```python
from build123d import *

# Parameters (mm, degrees)
SKETCH1_R           = 40
SKETCH1_R_2         = 25
BOSS_EXTRUDE1_DEPTH = 50
SKETCH2_R           = 2
CUT_EXTRUDE1_DEPTH  = 10
BOSS_EXTRUDE2_START = -30
BOSS_EXTRUDE2_DEPTH = 50


with BuildPart() as part:
    # Sketch1 → Boss-Extrude1 (new, symmetric)
    with BuildSketch(Plane(origin=(0, 0, 0), x_dir=(1, 0, 0), z_dir=(0, 1, 0))):
        with Locations(Location((0, 0, 0), (0, 0, 90))):
            Circle(SKETCH1_R)
        with Locations(Location((0, 0, 0), (0, 0, 90))):
            Circle(SKETCH1_R_2, mode=Mode.SUBTRACT)
    extrude(amount=BOSS_EXTRUDE1_DEPTH, both=True)

    # Sketch2 → Cut-Extrude1 (cut)
    with BuildSketch(Plane(origin=(0, 50, 0), x_dir=(1, 0, 0), z_dir=(0, 1, 0))):
        with Locations(Location((0, 35, 0), (0, 0, 270))):
            Circle(SKETCH2_R)
        with Locations(Location((35, 0, 0), (0, 0, 270))):
            Circle(SKETCH2_R)
        with Locations(Location((0, -35, 0), (0, 0, 270))):
            Circle(SKETCH2_R)
        with Locations(Location((-35, 0, 0), (0, 0, 270))):
            Circle(SKETCH2_R)
    cut_extrude1 = extrude(amount=-CUT_EXTRUDE1_DEPTH, mode=Mode.SUBTRACT)

    # Mirror1: Cut-Extrude1 across plane
    add(cut_extrude1.mirror(Plane.ZX), mode=Mode.SUBTRACT)

    # Sketch3 → Boss-Extrude2 (add)
    with BuildSketch(Plane.XZ.offset(50).offset(BOSS_EXTRUDE2_START)):
        with BuildLine():
            ThreePointArc((-5.985352508, 16.444620864), (-4.529333289, 16.90370196), (-3.038843109, 17.234135678))
            Line((-3.038843109, 17.234135678), (-4.341204442, 24.620193825))
            ThreePointArc((-4.341204442, 24.620193825), (-6.470476128, 24.148145657), (-8.550503583, 23.49231552))
            Line((-8.550503583, 23.49231552), (-5.985352508, 16.444620864))
        make_face()
        with BuildLine():
            Line((4.341204442, 24.620193825), (3.038843109, 17.234135678))
            ThreePointArc((3.038843109, 17.234135678), (4.529333289, 16.90370196), (5.985352508, 16.444620864))
            Line((5.985352508, 16.444620864), (8.550503583, 23.49231552))
            ThreePointArc((8.550503583, 23.49231552), (6.470476128, 24.148145657), (4.341204442, 24.620193825))
        make_face()
    boss_extrude2 = extrude(amount=-BOSS_EXTRUDE2_DEPTH)

    # Mirror2: Boss-Extrude2 across plane
    add(boss_extrude2.mirror(Plane.XY))


solid = part.part
```
Source: CAD feature listing. Evaluate the final solid. Frame: model axes, mm. A direction names the side the tool comes from. Round coordinates to 2 decimals unless told otherwise and drop trailing zeros. Write each loop counter-clockwise with the first axis right and the second up, starting at its lowest first coordinate (ties: lowest second). Pieces come first, ordered by that corner, then holes. Notation, with made-up numbers: M -3,81 L 47,81 A35 cw 47,120 Z; hole C 84.5,-26.5 d1. An arc over 180 degrees is marked long. Answer as a JSON object with one key per item and string values. Group by question number.
(1) Mould query, pull axis X, two halves, no side actions, for faces 1 (the flat face through (6, -20, -21)), 2 (the flat face through (-6, 30, -21)), 3 (the cylindrical face through (39.05, 0.7, 8.67)), 4 (the flat face through (-18.34, -50, -17.22)). Classes: +X half, -X half, draft (parallel to the pull), parting line (faces both ways), or undercut.
(2) Section query C-C on z = -22. Output: boundary loops of the cut face in (x, y), then the cut area to 3 significant figures.
(3) Section query A-A on x = 0. Output: boundary loops of the cut face in (y, z).
(4) First-contact query: pin 1 (4.5 mm diameter, centred on x = -35, z = 0, fed in from -Y); pin 2 (2.5 mm diameter, centred on x = 0, z = -35, fed in from +Y); pin 3 (3 mm diameter, centred on x = -17.5, y = -22.5, fed in from +Z); pin 4 (6 mm diameter, centred on x = -5.5, z = 19, fed in from -Y). Flat tips, straight axial feed; report the tip coordinate or a pass-through.
(5) Reachability of faces 5 (the flat face through (0, 40, -35)), 6 (the flat face through (-6, -20, 21)), 7 (the flat face through (7.25, 4.65, -19.92)) from +Z, -Z, +X, -X, +Y, -Y: full face, straight path, thin tool, end or side. Return the list, or none.
(6) Section query D-D on z = 11. Output: boundary loops of the cut face in (x, y), then the cut area to 3 significant figures.
(7) Section query B-B on y = 26. Output: boundary loops of the cut face in (x, z).
(8) Ray query, line 1 (X direction, y = -47, z = 0); line 2 (X direction, y = -7, z = -21); line 3 (Z direction, x = -1, y = 18). Return the intervals inside material, ascending. Write a range as [from, to].
Computed values:
{
 "1": {"face 1": "undercut", "face 2": "undercut", "face 3": "parting line", "face 4": "draft"},
 "2": {"outline": "M -33.41,-50 L -11.87,-50 L -11.87,50 L -33.41,50 Z; M -8.01,-20 L -3.88,-20 L -3.88,30 L -8.01,30 Z; M 3.88,-20 L 8.01,-20 L 8.01,30 L 3.88,30 Z; M 11.87,-50 L 33.41,-50 L 33.41,50 L 11.87,50 Z", "area": "4,720 mm^2"},
 "3": {"outline": "M -50,-40 L 50,-40 L 50,-37 L 40,-37 L 40,-33 L 50,-33 L 50,-25 L -50,-25 L -50,-33 L -40,-33 L -40,-37 L -50,-37 Z; M -50,25 L 50,25 L 50,33 L 40,33 L 40,37 L 50,37 L 50,40 L -50,40 L -50,37 L -40,37 L -40,33 L -50,33 Z"},
 "4": {"pin 1": "y = -50", "pin 2": "y = 40", "pin 3": "z = 36.66", "pin 4": "y = -20"},
 "5": {"face 5": "+Y", "face 6": "-Y", "face 7": "+Y, -Y"},
 "6": {"outline": "M -38.46,-50 L -22.45,-50 L -22.45,50 L -38.46,50 Z; M 22.45,-50 L 38.46,-50 L 38.46,50 L 22.45,50 Z", "area": "3,200 mm^2"},
 "7": {"outline": "C 0,0 d80; hole M -8.55,-23.49 L -5.99,-16.44 A17.5 ccw -3.04,-17.23 L -4.34,-24.62 A25 ccw 4.34,-24.62 L 3.04,-17.23 A17.5 ccw 5.99,-16.44 L 8.55,-23.49 A25 ccw 8.55,23.49 L 5.99,16.44 A17.5 ccw 3.04,17.23 L 4.34,24.62 A25 ccw -4.34,24.62 L -3.04,17.23 A17.5 ccw -5.99,16.44 L -8.55,23.49 A25 ccw Z"},
 "8": {"line 1": "[-40, -37], [-33, -25], [25, 33], [37, 40]", "line 2": "[-34.04, -13.56], [-7.64, -3.7], [3.7, 7.64], [13.56, 34.04]", "line 3": "[-39.99, -24.98], [24.98, 39.99]"}
}
